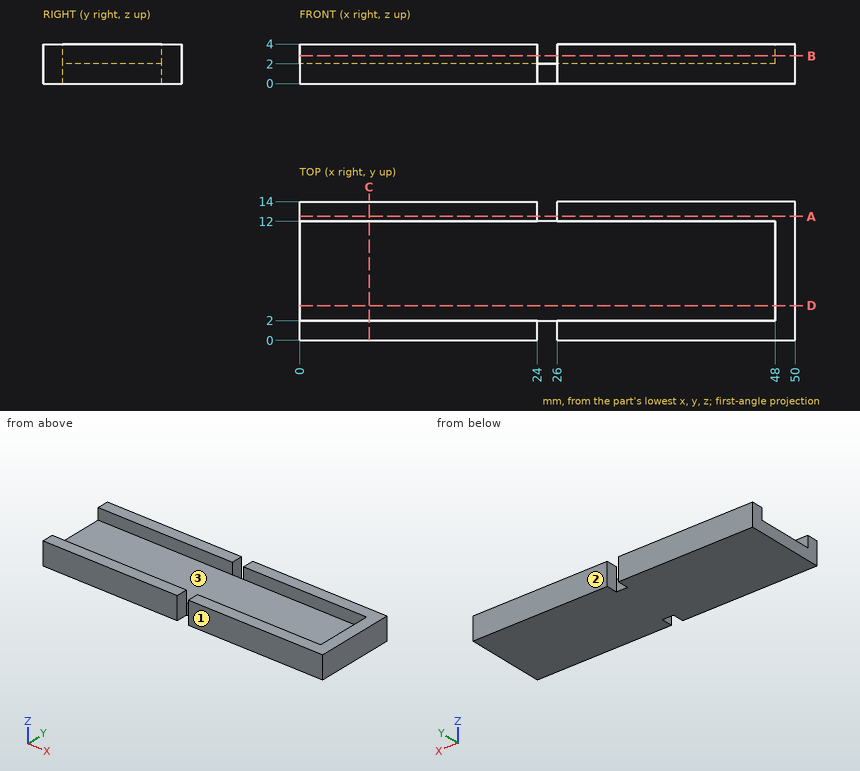
Source: three-view drawing plus pictorial views. Frame: mm from the lowest corner of the part. Give positions to 0.01 mm unless a question says otherwise; leave off trailing zeros. Order: outer loops, then holes, each group sorted by start corner. A loop starts at its lowest first (then second) coordinate and runs counter-clockwise, first axis right, second up. Notation, with made-up numbers: M 54.25,-37 L 86.25,-37 A25 ccw 86.25,-19 Z; hole C 76,-19.5 d6. An arc over 180 degrees is marked long. One line per question, with ' | ' between items.
1) Section D-D on y = 3.5. Output: boundary loops of the cut face in (x, z), and give its area (3 significant figures).
Filled in:
outline: M 0,0 L 50,0 L 50,4 L 48,4 L 48,2 L 0,2 Z | area: 104 mm2
2) Section A-A on y = 12.5. Output: boundary loops of the cut face in (x, z), and give its area (3 significant figures).
Filled in:
outline: M 0,0 L 24,0 L 24,4 L 0,4 Z; M 26,0 L 50,0 L 50,4 L 26,4 Z | area: 192 mm2
3) Contact query for flat-ended pins moving along their axis: P1, Ø1.5, axis at x = 19, y = 10, coming from the -Z side; P2, Ø1.6, axis at y = 5.5, z = 3.5, coming from the -X side; P3, Ø5, axis at x = 18.5, y = 5, coming from the +Z side. Output: stop coordinate, or through.
Filled in:
P1: stops at z = 0 | P2: stops at x = 48 | P3: stops at z = 2
4) Ray query, L1, parallel to Y at x = 45, z = 3.55; L2, parallel to X at y = 1, z = 2.55; L3, parallel to Z at x = 21.5, y = 8.25. Return the intervals inside material, ascending.
Filled in:
L1: y = 0 to 2, 12 to 14 | L2: x = 0 to 24, 26 to 50 | L3: z = 0 to 2
5) Section C-C on x = 7. Output: boundary loops of the cut face in (y, z), and give its area (3 significant figures).
Filled in:
outline: M 0,0 L 14,0 L 14,4 L 12,4 L 12,2 L 2,2 L 2,4 L 0,4 Z | area: 36.0 mm2
6) Section B-B on z = 2.8. Output: boundary loops of the cut face in (x, y), and give its area (3 significant figures).
Filled in:
outline: M 0,0 L 24,0 L 24,2 L 0,2 Z; M 0,12 L 24,12 L 24,14 L 0,14 Z; M 26,0 L 50,0 L 50,14 L 26,14 L 26,12 L 48,12 L 48,2 L 26,2 Z | area: 212 mm2
7) Draft query along Y for the marked faces 1, 2 and 3. Return one class per face: pulls with the +Y half, pulls with the -Y half, needs draft (parallel to the pull), parting line crosses it, or undercut.
Filled in:
face 1: pulls with the -Y half | face 2: pulls with the +Y half | face 3: undercut
